Here's how the part is built. I have some questions about the finished solid (model axes, mm). A direction names the side the tool comes from. Give positions to 0.01 mm unless a question says otherwise; leave off trailing zeros. Loops run counter-clockwise (first coordinate to the right, second up) from the corner with the lowest first, then second, coordinate; pieces in that order, holes last.
Q1. If we section it at C-C (z = 14): Please give me the cut outline in (x, y), plus the area to 3 significant figures.
Q2. For faces 1 (the face through (-1, 1, 3.048)), 2 (the face through (-1, -46.902, -2)), 3 (the face through (55.179, -1, 0)), 4 (the face through (1, -51.474, 38)), 5 (the face through (-55.179, -1, 0)), which set-ups out of +Z, -Z, +X, -X, +Y, -Y let a thin tool reach every point of the face, with its end or its side?
Q3. If we section it at A-A (x = -35): Please give me the cut outline in (y, z), plus the area to 3 significant figures.
Q4. Will these pins go through, and if not, where does the flat tip stop? P1, Ø1.8, axis at y = -3.5, z = -1, coming from the +X side; P2, Ø6, axis at x = -18.5, y = 34.5, coming from the +Z side; P3, Ø1.5, axis at x = 7.5, z = 56.5, coming from the +Y side; P4, Ø5, axis at x = 8, y = -48.5, coming from the -Z side.
Q5. I need wall thicknesses on line 1 (Z direction, x = 40, y = 42.5); line 2 (X direction, y = 16.5, z = 1); line 3 (Y direction, x = 0, z = 14). Which ranges of each line are inside material? Lowest first, please.
Q6. If we section it at B-B (y = 31): Please give me the cut outline in (x, z), plus the area to 3 significant figures.
from build123d import *

# Parameters (mm, degrees)
F0_W     = 110.358618
F0_H     = 93.804828
F3_DEPTH = 3.048
F2_W     = 113.771484
F2_H     = 74.878134
F4_DEPTH = 4.572


with BuildPart() as f3:
    # F0 (on Top) → F3 (new body, symmetric)
    with BuildSketch(Plane.XY):
        Rectangle(F0_W, F0_H)
    extrude(amount=F3_DEPTH, both=True)

    # F2 (on face) → F4 (join)
    with BuildSketch(Plane.XZ.offset(46.902414)):
        with Locations((1.378391, 37.439067)):
            Rectangle(F2_W, F2_H)
    extrude(amount=F4_DEPTH)


solid = f3.part
Check sheet entries:
1. outline: (-55.51, -51.47) - (58.26, -51.47) - (58.26, -46.9) - (-55.51, -46.9) - close
1. area: 520 mm2
2. face 1: +Z, +X, -X, +Y
2. face 2: -Z, +X, -X, -Y
2. face 3: +Z, -Z, +X, +Y
2. face 4: +Z, -Z, +X, -X, -Y
2. face 5: +Z, -Z, -X, +Y
3. outline: (-51.47, 0) - (-46.9, 0) - (-46.9, -3.05) - (46.9, -3.05) - (46.9, 3.05) - (-46.9, 3.05) - (-46.9, 74.88) - (-51.47, 74.88) - close
3. area: 914 mm2
4. P1: stops at x = 55.18
4. P2: stops at z = 3.05
4. P3: stops at y = -46.9
4. P4: stops at z = -3.05
5. line 1: z = -3.05 to 3.05
5. line 2: x = -55.18 to 55.18
5. line 3: y = -51.47 to -46.9
6. outline: (-55.18, -3.05) - (55.18, -3.05) - (55.18, 3.05) - (-55.18, 3.05) - close
6. area: 673 mm2
